Read the model definition and answer for the solid it produces. Units are mm, in the model's axes. A direction names the side the tool comes from. Coordinates: 2 decimals unless noted, no trailing zeros. Write each loop counter-clockwise with the first axis right and the second up, starting at its lowest first coordinate (ties: lowest second). Pieces come first, ordered by that corner, then holes.
from build123d import *

# Parameters (mm, degrees)
SKETCH_R        = 1.95
PAD_DEPTH       = 26
SKETCH002_W     = 18
SKETCH002_H     = 22
POCKET_DEPTH    = 20.05
SKETCH003_W     = 18.7
SKETCH003_H     = 19.57
POCKET001_DEPTH = 1.5
CHAMFER_SIZE    = 0.5
SKETCH004_R     = 0.8
POCKET002_DEPTH = 4


with BuildPart() as part:
    # Sketch → Pad (new body)
    with BuildSketch(Plane.XY):
        with BuildLine():
            Line((14, 9.5), (16, 9.5))
            Line((16, 9.5), (16, -9.5))
            Line((16, -9.5), (14, -9.5))
            Line((14, -9.5), (14, -8.5))
            Line((0, -4), (14, -8.5))
            ThreePointArc((0, 4), (-4, 0), (0, -4))
            Line((0, 4), (14, 8.5))
            Line((14, 8.5), (14, 9.5))
        make_face()
        Circle(SKETCH_R, mode=Mode.SUBTRACT)
        Polygon((4, 1.75), (4, -1.75), (14, -5.5), (14, 5.5), align=None, mode=Mode.SUBTRACT)
    extrude(amount=PAD_DEPTH)

    # Sketch002 (on Face14 of Pad) → Pocket (cut)
    with BuildSketch(Plane(origin=(0, 0, 0), x_dir=(1, 0, 0), z_dir=(0, 0, -1))):
        with Locations((3, 0)):
            Rectangle(SKETCH002_W, SKETCH002_H)
    extrude(amount=-POCKET_DEPTH, mode=Mode.SUBTRACT)

    # Sketch003 (on Face6 of Pocket) → Pocket001 (cut)
    with BuildSketch(Plane.XY.offset(26)):
        with Locations((2.65, 0.635)):
            Rectangle(SKETCH003_W, SKETCH003_H)
    extrude(amount=-POCKET001_DEPTH, mode=Mode.SUBTRACT)

    # Chamfer
    chamfer_edges = [part.edges().sort_by_distance(p)[0] for p in [
        (6, -5.928571, 20.05),
        (-4, 0, 20.05),
        (6, 5.928571, 20.05),
        (12, 6.303571, 20.05),
        (8, 3.25, 20.05),
        (4, 0, 20.05),
        (8, -3.25, 20.05),
        (12, -6.303571, 20.05),
        (-1.95, 0, 20.05),
        (12, 6.303571, 26),
        (12, 4.75, 25.25),
        (12, 6.303571, 24.5),
        (12, 7.857143, 25.25),
        (6, 5.928571, 24.5),
        (-4, 0, 24.5),
        (6, -5.928571, 24.5),
        (12, -6.303571, 24.5),
        (8, -3.25, 24.5),
        (4, 0, 24.5),
        (8, 3.25, 24.5),
        (-1.95, 0, 24.5),
        (12, -6.303571, 26),
        (12, -7.857143, 25.25),
        (12, -4.75, 25.25),
        (12, 6.303571, 0),
        (12, 7.857143, 10.025),
        (12, 4.75, 10.025),
        (12, -6.303571, 0),
        (12, -4.75, 10.025),
        (12, -7.857143, 10.025),
    ]]
    chamfer(chamfer_edges, length=CHAMFER_SIZE)

    # Sketch004 (on Face20 of Chamfer) → Pocket002 (cut)
    with BuildSketch(Plane.YZ.offset(16)):
        with Locations((7, 23.5)):
            Circle(SKETCH004_R)
        with Locations((7, 2.5)):
            Circle(SKETCH004_R)
        with Locations((-7, 2.5)):
            Circle(SKETCH004_R)
        with Locations((-7, 23.5)):
            Circle(SKETCH004_R)
    extrude(amount=-POCKET002_DEPTH, mode=Mode.SUBTRACT)


solid = part.part
Item 1: Given pin 1 (1 mm diameter, centred on y = 7, z = 23.5, fed in from +X); pin 2 (0.6 mm diameter, centred on y = -6.5, z = 7.5, fed in from -X); pin 3 (2 mm diameter, centred on x = 9.5, y = 1.5, fed in from -Z); pin 4 (7 mm diameter, centred on x = 2, y = 2, fed in from -Z), each flat-ended and moving along its own axis, determine where each tip first touches the part or whether it passes through.
Item 2: The part is cut by section C-C (x = 6). Give the vertices of the cut face in (y, z).
Item 3: The part is cut by section A-A (y = 0). Give the vertices of the cut face in (x, z).
Item 4: The part is cut by section D-D (x = 14.5). Give the vertices of the cut face in (y, z), and give its area (3 significant figures).
Item 5: The part is cut by section B-B (z = 23.5). Give the vertices of the cut face in (x, y), and give its area (3 significant figures).
Item 6: Determine the mould class of faces 6 (the flat face through (12, 7, 24)), 7 (the cylindrical face through (14.028, -6.261, 2.194)), 8 (the flat face through (15, 0, 26)), 9 (the cylindrical face through (-4, 0, 22)) for opening direction Z: +Z half, -Z half, draft (parallel to the pull), parting line (faces both ways), or undercut.
Item 7: Find the intervals of material crossed by probe 1 along Y at (x, z) = (14.95, 2.5); probe 2 along X at (y, z) = (0, 22.55); probe 3 along Z at (x, y) = (13.65, 7), in increasing order.
Item 8: For faces 1 (the flat face through (12, -7, 24)), 2 (the flat face through (12.68, -5.005, 17.754)), 3 (the flat face through (7.53, 3.34, 20.3)), 4 (the flat face through (14, 9, 13)), 5 (the flat face through (12, 6, 10)), determine the directions among +Z, -Z, +X, -X, +Y, -Y from which every point of the face is accessible in a straight line to the end or side of a thin tool.
Answer:
1. pin 1: stops at x = 12
1. pin 2: stops at x = 12
1. pin 3: passes through
1. pin 4: stops at z = 20.05
2. outline: (-5.93, 20.55) - (-5.4, 20.05) - (-3.03, 20.05) - (-2.5, 20.55) - (-2.5, 24) - (-3.03, 24.5) - (-5.4, 24.5) - (-5.93, 24) - close; (2.5, 20.55) - (3.03, 20.05) - (5.4, 20.05) - (5.93, 20.55) - (5.93, 24) - (5.4, 24.5) - (3.03, 24.5) - (2.5, 24) - close
3. outline: (-4, 20.55) - (-3.5, 20.05) - (-2.45, 20.05) - (-1.95, 20.55) - (-1.95, 24) - (-2.45, 24.5) - (-3.5, 24.5) - (-4, 24) - close; (1.95, 20.55) - (2.45, 20.05) - (3.5, 20.05) - (4, 20.55) - (4, 24) - (3.5, 24.5) - (2.45, 24.5) - (1.95, 24) - close; (14, 0) - (16, 0) - (16, 26) - (14, 26) - close
4. outline: (-9.5, 0) - (9.5, 0) - (9.5, 26) - (-9.5, 26) - close; hole circle Ø1.6 at (-7, 2.5); hole circle Ø1.6 at (-7, 23.5); hole circle Ø1.6 at (7, 2.5); hole circle Ø1.6 at (7, 23.5)
4. area: 486 mm2
5. outline: (0, -4) - (14, -8.5) - (14, -9.5) - (16, -9.5) - (16, -7.8) - (12, -7.8) - (12, -6.2) - (16, -6.2) - (16, 6.2) - (12, 6.2) - (12, 7.8) - (16, 7.8) - (16, 9.5) - (14, 9.5) - (14, 8.5) - (0, 4) arc R4 ccw to start; hole circle Ø3.9 at (0, 0); hole (4, -1.75) - (14, -5.5) - (14, 5.5) - (4, 1.75) - close
5. area: 141 mm2
6. face 6: undercut
6. face 7: undercut
6. face 8: +Z half
6. face 9: draft
7. probe 1: y = -9.5 to -7.8, -6.2 to 6.2, 7.8 to 9.5
7. probe 2: x = -4 to -1.95, 1.95 to 4, 14 to 16
7. probe 3: z = 0 to 1.7, 3.3 to 22.7, 24.3 to 26
8. face 1: +X
8. face 2: +Z, -Z
8. face 3: -Z
8. face 4: +Z, -Z, -X, +Y
8. face 5: -Z, -X, +Y, -Y
